from build123d import *

# Parameters (mm, degrees)
F0_W      = 21
F0_H      = 114
F1_DEPTH  = 65
F2_W      = 19
F2_H      = 112
F3_DEPTH  = 90
F4_W      = 10
F4_H      = 4
F5_DEPTH  = 25
F6_W      = 114
F6_H      = 1
F7_DEPTH  = 1
F8_W      = 114
F8_H      = 1
F9_DEPTH  = 1
F11_DEPTH = 25
F12_W     = 20
F12_H     = 6
F13_DEPTH = 0.5
F15_DEPTH = 25


with BuildPart() as f1:
    # F0 (on Top) → F1 (new body)
    with BuildSketch(Plane.XY):
        Rectangle(F0_W, F0_H)
    extrude(amount=F1_DEPTH)

    # F2 (on face) → F3 (cut)
    with BuildSketch(Plane.XY.offset(65)):
        Rectangle(F2_W, F2_H)
    extrude(amount=-F3_DEPTH, mode=Mode.SUBTRACT)

    # F4 (on face) → F5 (cut)
    with BuildSketch(Plane.XZ.offset(57)):
        with Locations((0, 46)):
            Rectangle(F4_W, F4_H)
    extrude(amount=-F5_DEPTH, mode=Mode.SUBTRACT)

    # F6 (on face) → F7 (join)
    with BuildSketch(Plane.YZ.offset(10.5)):
        with Locations((0, 0.5)):
            Rectangle(F6_W, F6_H)
    extrude(amount=F7_DEPTH)

    # F8 (on face) → F9 (join)
    with BuildSketch(Plane(origin=(-10.5, 0, 0), x_dir=(0, -1, 0), z_dir=(-1, 0, 0))):
        with Locations((0, 0.5)):
            Rectangle(F8_W, F8_H)
    extrude(amount=F9_DEPTH)

    # F10 (on face) → F11 (cut)
    with BuildSketch(Plane.YZ.offset(10.5)):
        with BuildLine():
            ThreePointArc((43, 65), (52.899495, 60.899495), (57, 51))
            Line((57, 51), (57, 65))
            Line((57, 65), (43, 65))
        make_face()
    extrude(amount=-F11_DEPTH, mode=Mode.SUBTRACT)

    # F12 (on face) → F13 (join)
    with BuildSketch(Plane(origin=(0, 57, 0), x_dir=(-1, 0, 0), z_dir=(0, 1, 0))):
        with Locations((0, 48)):
            Rectangle(F12_W, F12_H)
    extrude(amount=F13_DEPTH)

    # F14 (on face) → F15 (cut)
    with BuildSketch(Plane(origin=(-10, 0, 0), x_dir=(0, -1, 0), z_dir=(-1, 0, 0))):
        Polygon((-57.5, 51), (-57.5, 48), (-57, 51), align=None)
    extrude(amount=-F15_DEPTH, mode=Mode.SUBTRACT)


solid = f1.part
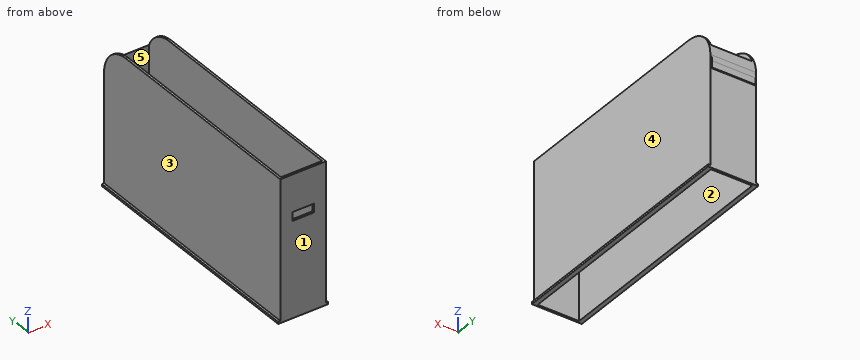
Read the model definition and answer for the solid it produces. Units are mm, in the model's axes. Face numbers are marked on the shaded views. A direction names the side the tool comes from. Coordinates: 2 decimals unless noted, no trailing zeros. Order: outer loops, then holes, each group sorted by start corner. A loop starts at its lowest first (then second) coordinate and runs counter-clockwise, first axis right, second up. Notation, with made-up numbers: (-14.75, 1) -> (11.25, 1) arc R9 cw to (11.25, 8) -> close; hole circle Ø2 at (61, -20). An arc over 180 degrees is marked (long way). Answer as a JSON object with one key per item and string values.
1) Consider line 1 along X through (y, z) = (-20, 8.5); line 2 along Y through (x, z) = (-2, 11); line 3 along Y through (x, z) = (-4.5, 54). Determine where each line is inside the solid, lowest interval first. Write a range as from..to.
Model answer:
{"line 1": "x = -10.5..-9.5, 9.5..10.5", "line 2": "y = -57..-56, 56..57", "line 3": "y = -57..-56, 56..56.67"}
2) A cutting plane is placed at B-B, the plane y = 39. Determine the outline of the cut face in (x, z), plus the area to 3 significant figures.
Model answer:
{"outline": "(-11.5, 0) -> (-9.5, 0) -> (-9.5, 65) -> (-10.5, 65) -> (-10.5, 1) -> (-11.5, 1) -> close; (9.5, 0) -> (11.5, 0) -> (11.5, 1) -> (10.5, 1) -> (10.5, 65) -> (9.5, 65) -> close", "area": "132 mm²"}
3) A cutting plane is placed at C-C, the plane z = 11.5. Determine the outline of the cut face in (x, y).
Model answer:
{"outline": "(-10.5, -57) -> (10.5, -57) -> (10.5, 57) -> (-10.5, 57) -> close; hole (-9.5, -56) -> (9.5, -56) -> (9.5, 56) -> (-9.5, 56) -> close"}
4) The mould has two halves that part along Y. Classify the marked faces 1, 2 and 3: released by +Y, released by -Y, zero draft, split by the parting line, or undercut.
Model answer:
{"face 1": "released by -Y", "face 2": "undercut", "face 3": "zero draft"}
5) Each of these flat-tipped pins is pushed along its axis until it touches: pin 1 (0.5 mm diameter, centred on x = 1.5, y = -56.5, fed in from -Z); pin 2 (3 mm diameter, centred on y = -15.5, z = 33.5, fed in from -X); pin 3 (5 mm diameter, centred on x = 7.5, z = 53, fed in from +Y); pin 4 (12 mm diameter, centred on x = -2, z = 14, fed in from +Y). Where does it stop, or does it pass through?
Model answer:
{"pin 1": "stops at z = 0", "pin 2": "stops at x = -10.5", "pin 3": "stops at y = 57.08", "pin 4": "stops at y = 57"}
6) A cutting plane is placed at A-A, the plane x = 6.5. Determine the outline of the cut face in (y, z).
Model answer:
{"outline": "(-57, 0) -> (-56, 0) -> (-56, 65) -> (-57, 65) -> close; (56, 0) -> (57, 0) -> (57, 45) -> (57.5, 45) -> (57.5, 48) -> (57, 51) arc R14 ccw to (56, 56.2) -> close"}
7) A tool of negligible diameter and unlimited length cuts with its end or side. For the marked faces 4 and 5, from which of +Z, -Z, +X, -X, +Y, -Y can it reach the whole face along a straight path? Write none if from no direction.
Model answer:
{"face 4": "+Z, +X, +Y, -Y", "face 5": "+Z, -Z"}
